Could you check a few things on this model? Use its own coordinates, in mm. A direction names the side the tool comes from. Round coordinates to 2 decimals unless told otherwise and drop trailing zeros. Order: outer loops, then holes, each group sorted by start corner. A loop starts at its lowest first (then second) coordinate and runs counter-clockwise, first axis right, second up. Notation, with made-up numbers: (4, 59) - (61, 59) arc R24 ccw to (61, 79) - close; hole circle Ø9 at (68.25, -34). An arc over 180 degrees is marked (long way). Use one line per item in the form item = value.
from build123d import *

# Parameters (mm, degrees)
BOSS_EXTRUDE1_DEPTH = 40
SHELL1_T            = -4
SKETCH4_R           = 1.5
CUT_EXTRUDE1_DEPTH  = 40
SKETCH6_R           = 3.5
BOSS_EXTRUDE2_DEPTH = 40
SKETCH7_R           = 6
BOSS_EXTRUDE3_DEPTH = 30
SKETCH11_R          = 7.621273112
CUT_EXTRUDE2_DEPTH  = 10
SKETCH14_W          = 5.073937662
SKETCH14_H          = 24.893505848
BOSS_EXTRUDE5_DEPTH = 57
SKETCH15_R          = 2.42948244
CUT_EXTRUDE4_DEPTH  = 57
SKETCH18_R          = 94.524667443
SKETCH18_R_2        = 90.107612794
BOSS_EXTRUDE7_DEPTH = 72


with BuildPart() as part:
    # Sketch2 → Boss-Extrude1 (new body)
    with BuildSketch(Plane(origin=(0, 0, 0), x_dir=(0, 0, -1), z_dir=(1, 0, 0))):
        with BuildLine():
            ThreePointArc((42.291021672, 3.859649123), (27.646360731, -31.495689937), (-7.708978328, -46.140350877))
            Line((-7.708978328, -46.140350877), (242.291021672, -46.140350877))
            ThreePointArc((242.291021672, -46.140350877), (192.291021672, 3.859649123), (242.291021672, 53.859649123))
            Line((242.291021672, 53.859649123), (-7.708978328, 53.859649123))
            ThreePointArc((-7.708978328, 53.859649123), (27.646360731, 39.214988182), (42.291021672, 3.859649123))
        make_face()
        with BuildLine():
            ThreePointArc((-7.708978328, 53.859649123), (-57.708978328, 3.859649123), (-7.708978328, -46.140350877))
            Line((-7.708978328, -46.140350877), (-7.708978328, 53.859649123))
        make_face()
        with BuildLine():
            Line((-7.708978328, 53.859649123), (-7.708978328, -46.140350877))
            ThreePointArc((-7.708978328, -46.140350877), (27.646360731, -31.495689937), (42.291021672, 3.859649123))
            ThreePointArc((42.291021672, 3.859649123), (27.646360731, 39.214988182), (-7.708978328, 53.859649123))
        make_face()
        with BuildLine():
            ThreePointArc((242.291021672, 53.859649123), (192.291021672, 3.859649123), (242.291021672, -46.140350877))
            Line((242.291021672, -46.140350877), (242.291021672, 53.859649123))
        make_face()
        with BuildLine():
            Line((242.291021672, 53.859649123), (242.291021672, -46.140350877))
            ThreePointArc((242.291021672, -46.140350877), (277.646360731, -31.495689937), (292.291021672, 3.859649123))
            ThreePointArc((292.291021672, 3.859649123), (277.646360731, 39.214988182), (242.291021672, 53.859649123))
        make_face()
    extrude(amount=BOSS_EXTRUDE1_DEPTH)

    # Shell1
    shell1_openings = [part.faces().sort_by_distance(p)[0] for p in [
        (0, 3.859649123, -117.291021672),
    ]]
    offset(amount=SHELL1_T, openings=shell1_openings, kind=Kind.INTERSECTION)

    # Sketch4 → Cut-Extrude1 (cut)
    with BuildSketch(Plane.ZY.offset(-36)):
        with Locations((-252.791021672, 22.046182602)):
            Circle(SKETCH4_R)
        with Locations((-231.791021672, 22.046182602)):
            Circle(SKETCH4_R)
        with Locations((-263.291021672, 3.859649123)):
            Circle(SKETCH4_R)
        with Locations((-221.291021672, 3.859649123)):
            Circle(SKETCH4_R)
        with Locations((-252.791021672, -14.326884357)):
            Circle(SKETCH4_R)
        with Locations((-231.791021672, -14.326884357)):
            Circle(SKETCH4_R)
    extrude(amount=-CUT_EXTRUDE1_DEPTH, mode=Mode.SUBTRACT)

    # Sketch6 → Boss-Extrude2 (add)
    with BuildSketch(Plane.ZY.offset(-36)):
        with Locations((-242.291021672, 3.859649123)):
            Circle(SKETCH6_R)
    extrude(amount=-BOSS_EXTRUDE2_DEPTH)

    # Sketch7 → Boss-Extrude3 (add)
    with BuildSketch(Plane(origin=(76, 0, 0), x_dir=(0, 0, -1), z_dir=(1, 0, 0))):
        with Locations((242.291021672, 3.859649123)):
            Circle(SKETCH7_R)
    extrude(amount=BOSS_EXTRUDE3_DEPTH)

    # Sketch11 → Cut-Extrude2 (cut)
    with BuildSketch(Plane(origin=(40, 0, 0), x_dir=(0, 0, -1), z_dir=(1, 0, 0))):
        Circle(SKETCH11_R)
    extrude(amount=-CUT_EXTRUDE2_DEPTH, mode=Mode.SUBTRACT)

    # Sketch14 → Boss-Extrude5 (add)
    with BuildSketch(Plane(origin=(40, 0, 0), x_dir=(0, 0, -1), z_dir=(1, 0, 0))):
        with Locations((97.267454621, -32.353135016)):
            Rectangle(SKETCH14_W, SKETCH14_H)
    extrude(amount=BOSS_EXTRUDE5_DEPTH)

    # Sketch15 → Cut-Extrude4 (cut)
    with BuildSketch(Plane(origin=(0, 0, -99.804423452), x_dir=(-1, 0, 0), z_dir=(0, 0, -1))):
        with Locations((-76.430932939, -32.204980858)):
            Circle(SKETCH15_R)
    extrude(amount=-CUT_EXTRUDE4_DEPTH, mode=Mode.SUBTRACT)

    # Sketch18 → Boss-Extrude7 (add)
    with BuildSketch(Plane(origin=(40, 0, 0), x_dir=(0, 0, -1), z_dir=(1, 0, 0))):
        with Locations(Location((25.75, 0, 0), (0, 0, 34.735906814))):
            Circle(SKETCH18_R)
        with Locations(Location((25.75, 0, 0), (0, 0, 36.707196429))):
            Circle(SKETCH18_R_2, mode=Mode.SUBTRACT)
    extrude(amount=BOSS_EXTRUDE7_DEPTH)


solid = part.part
Item 1: Imagine slicing it at D-D on z = -166. Please give me the cut outline in (x, y).
Found:
outline = (0, -46.14) - (40, -46.14) - (40, 53.86) - (0, 53.86) - (0, 49.86) - (36, 49.86) - (36, -42.14) - (0, -42.14) - close
Item 2: Imagine slicing it at C-C on y = 62. Please give me the cut outline in (x, z), plus the area to 3 significant figures.
Found:
outline = (40, -97.1) - (112, -97.1) - (112, -91.14) - (40, -91.14) - close; (40, 39.64) - (112, 39.64) - (112, 45.6) - (40, 45.6) - close
area = 859 mm2
Item 3: If we mould it in two halves opening along Z, with no side actions, what happens to faces 6 (the face through (19.72, 4.959, 57.697)), 7 (the face through (40, 6.2, 64.3)), 8 (the face through (38.03, -2.92, -7.04))? For each: released by +Z, released by -Z, zero draft, split by the parting line, or undercut.
Found:
face_6 = released by +Z
face_7 = zero draft
face_8 = undercut
Item 4: Imagine slicing it at B-B on x = 84. Please give me the cut outline in (y, z).
Found:
outline = circle Ø189.05 at (0, -25.75); (-44.8, -99.8) - (-19.91, -99.8) - (-19.91, -94.73) - (-44.8, -94.73) - close; circle Ø12 at (3.86, -242.29); hole circle Ø180.22 at (0, -25.75)
Item 5: I need wall thicknesses on L1, parallel to Y at x = 8, z = -6.5; L2, parallel to Y at x = 42.5, z = -98; L3, parallel to Y at x = 37, z = 0. Which ranges of each line are inside material? Lowest first, please.
Found:
L1 = -46.14 to -42.14, 49.86 to 53.86
L2 = -60.95 to -53.85, -44.8 to -19.91, 53.85 to 60.95
L3 = -46.14 to -7.62, 7.62 to 53.86
Item 6: For faces 1 (the face through (75.5, 73.07, -78.48)), 2 (the face through (36, 5, -120)), 3 (the face through (112, -49, -102)), 4 (the face through (106, 4, -242)), 5 (the face through (76, 1, -245)), which set-ups out of +Z, -Z, +X, -X, +Y, -Y let a thin tool reach every point of the face, with its end or its side?
Found:
face_1 = +X
face_2 = -X
face_3 = +Z, -Z, +X, +Y, -Y
face_4 = -Z, +X, +Y, -Y
face_5 = none
Item 7: Imagine slicing it at A-A on z = -25.75. Please give me the cut outline in (x, y).
Found:
outline = (0, -46.14) - (40, -46.14) - (40, 53.86) - (0, 53.86) - (0, 49.86) - (36, 49.86) - (36, -42.14) - (0, -42.14) - close; (40, -94.52) - (112, -94.52) - (112, -90.11) - (40, -90.11) - close; (40, 90.11) - (112, 90.11) - (112, 94.52) - (40, 94.52) - close
Item 8: Will these pins go through, and if not, where does the flat tip stop? P1, Ø5, axis at x = 30.5, y = 24, coming from the -Z side; P2, Ø3, axis at x = 76.43, y = -32.2, coming from the -Z side; P3, Ø2.5, axis at y = -30.5, z = -97, coming from the +X side; P4, Ø2.5, axis at y = 3.86, z = -221.29, coming from the -X side.
Found:
P1 = -289.08
P2 = -115.15
P3 = 97
P4 = through
